Autodesk Inventor part; units mm, degrees
ref_plane "YZ Plane" through (0, 0, 0) normal (1, 0, 0) x (0, 1, 0)
ref_plane "XZ Plane" through (0, 0, 0) normal (0, 1, 0) x (-1, 0, 0)
ref_plane "XY Plane" through (0, 0, 0) normal (0, 0, 1) x (1, 0, 0)
sketch "Sketch1" plane through (0, 0, 0) normal (0, 0, 1) x (1, 0, 0)
  arc A0 (-5.217, 1.3451) -> (-5.1032, 1.1142) centre (-4.8204, 1.397) ccw
  line L0 (-5.1032, 1.1142) -> (-4.8872, 0.8982)
  arc A1 (-4.77, 0.6153) -> (-4.8872, 0.8982) centre (-5.17, 0.6153) ccw
  line L1 (-4.77, 0.6153) -> (-4.77, -0.9467)
  arc A2 (-4.8872, -1.2296) -> (-4.77, -0.9467) centre (-5.17, -0.9467) ccw
  line L2 (-4.8872, -1.2296) -> (-7.2071, -3.5495)
  arc A3 (-7.2071, -3.5495) -> (-7.5, -4.2566) centre (-6.5, -4.2566) ccw
  line L3 (-7.5, -4.2566) -> (-7.5, -6.8)
  line L4 (-7.5, -6.8) -> (-6.8, -7.5)
  line L5 (-6.8, -7.5) -> (6.8, -7.5)
  line L6 (6.8, -7.5) -> (7.5, -6.8)
  line L7 (7.5, -6.8) -> (7.5, -4.2566)
  arc A4 (7.5, -4.2566) -> (7.2071, -3.5495) centre (6.5, -4.2566) ccw
  line L8 (7.2071, -3.5495) -> (4.8872, -1.2296)
  arc A5 (4.77, -0.9467) -> (4.8872, -1.2296) centre (5.17, -0.9467) ccw
  line L9 (4.77, -0.9467) -> (4.77, 0.6153)
  arc A6 (4.8872, 0.8982) -> (4.77, 0.6153) centre (5.17, 0.6153) ccw
  line L10 (4.8872, 0.8982) -> (5.1032, 1.1142)
  arc A7 (5.1032, 1.1142) -> (5.217, 1.3451) centre (4.8204, 1.397) ccw
  arc A8 (6.7419, 2.7529) -> (5.217, 1.3451) centre (6.8233, 1.1349) ccw
  line L11 (6.7419, 2.7529) -> (7.5, 3.511)
  line L12 (7.5, 3.511) -> (7.5, 5.049)
  line L13 (7.5, 5.049) -> (6.7304, 5.8186)
  arc A9 (5.2183, 7.2157) -> (6.7304, 5.8186) centre (6.8233, 7.436) ccw
  arc A10 (5.2183, 7.2157) -> (5.1049, 7.4441) centre (4.822, 7.1613) ccw
  line L14 (5.1049, 7.4441) -> (5.049, 7.5)
  line L15 (5.049, 7.5) -> (-5.049, 7.5)
  line L16 (-5.049, 7.5) -> (-5.1049, 7.4441)
  arc A11 (-5.1049, 7.4441) -> (-5.2183, 7.2157) centre (-4.822, 7.1613) ccw
  arc A12 (-6.7304, 5.8186) -> (-5.2183, 7.2157) centre (-6.8233, 7.436) ccw
  line L17 (-6.7304, 5.8186) -> (-7.5, 5.049)
  line L18 (-7.5, 5.049) -> (-7.5, 3.511)
  line L19 (-7.5, 3.511) -> (-6.7419, 2.7529)
  arc A13 (-5.217, 1.3451) -> (-6.7419, 2.7529) centre (-6.8233, 1.1349) ccw
  line L20 (-7.5, -5.5283) -> (-10, -5.5283)
  line L21 (-10, -5.5283) -> (-10, 14.2)
  line L22 (-10, 14.2) -> (10, 14.2)
  line L23 (10, 14.2) -> (10, -5.5283)
  line L24 (10, -5.5283) -> (7.5, -5.5283)
  arc A14 (-7.2778, -3.4788) -> (-7.6, -4.2566) centre (-6.5, -4.2566) ccw
  line L25 (-7.2778, -3.4788) -> (-4.9579, -1.1589)
  arc A15 (-4.9579, -1.1589) -> (-4.87, -0.9467) centre (-5.17, -0.9467) ccw
  line L26 (-4.87, -0.9467) -> (-4.87, 0.6153)
  arc A16 (-4.87, 0.6153) -> (-4.9579, 0.8275) centre (-5.17, 0.6153) ccw
  line L27 (-4.9579, 0.8275) -> (-5.1739, 1.0435)
  arc A17 (-5.3161, 1.3322) -> (-5.1739, 1.0435) centre (-4.8204, 1.397) ccw
  arc A18 (-5.3161, 1.3322) -> (-6.7848, 2.6544) centre (-6.8233, 1.1349) ccw
  line L28 (-6.7848, 2.6544) -> (-7.6, 3.4696)
  line L29 (-7.6, 3.4696) -> (-7.6, 5.0904)
  line L30 (-7.6, 5.0904) -> (-6.7736, 5.9168)
  arc A19 (-6.7736, 5.9168) -> (-5.3174, 7.2293) centre (-6.8233, 7.436) ccw
  arc A20 (-5.1756, 7.5148) -> (-5.3174, 7.2293) centre (-4.822, 7.1613) ccw
  line L31 (-5.1756, 7.5148) -> (-5.0904, 7.6)
  line L32 (-5.0904, 7.6) -> (5.0904, 7.6)
  line L33 (5.0904, 7.6) -> (5.1756, 7.5148)
  arc A21 (5.3174, 7.2293) -> (5.1756, 7.5148) centre (4.822, 7.1613) ccw
  arc A22 (5.3174, 7.2293) -> (6.7736, 5.9168) centre (6.8233, 7.436) ccw
  line L34 (6.7736, 5.9168) -> (7.6, 5.0904)
  line L35 (7.6, 5.0904) -> (7.6, 3.4696)
  line L36 (7.6, 3.4696) -> (6.7848, 2.6544)
  arc A23 (6.7848, 2.6544) -> (5.3161, 1.3322) centre (6.8233, 1.1349) ccw
  arc A24 (5.1739, 1.0435) -> (5.3161, 1.3322) centre (4.8204, 1.397) ccw
  line L37 (5.1739, 1.0435) -> (4.9579, 0.8275)
  arc A25 (4.9579, 0.8275) -> (4.87, 0.6153) centre (5.17, 0.6153) ccw
  line L38 (4.87, 0.6153) -> (4.87, -0.9467)
  arc A26 (4.87, -0.9467) -> (4.9579, -1.1589) centre (5.17, -0.9467) ccw
  line L39 (4.9579, -1.1589) -> (7.2778, -3.4788)
  arc A27 (7.6, -4.2566) -> (7.2778, -3.4788) centre (6.5, -4.2566) ccw
  line L40 (7.6, -4.2566) -> (7.6, -6.8414)
  line L41 (7.6, -6.8414) -> (6.8414, -7.6)
  line L42 (6.8414, -7.6) -> (-6.8414, -7.6)
  line L43 (-6.8414, -7.6) -> (-7.6, -6.8414)
  line L44 (-7.6, -6.8414) -> (-7.6, -4.2566)
  point P0 (0, 0)
  point P1 (-7.6, -5.5283)
  point P2 (7.6, -5.5283)
  dimension "d2" = 6.7
  dimension "d20" = 2.5
  dimension "d21" = 0.1
extrude "Extrusion1" add sketch "Sketch1" against normal blind 15 contours L20 L21 L22 L23 L24 L40 A27 L39 A26 L38 A25 L37 A24 A23 L36 L35 L34 A22 A21 L33 L32 L31 A20 A19 L30 L29 L28 A18 A17 L27 A16 L26 A15 L25 A14 L44
chamfer "Chamfer1" distance 1.5 angle 45 10 edges at (-10, -5.5283, -7.5) (-10, 4.3358, -15) (-10, 4.3358, 0) (0, 14.2, -15) (0, 14.2, 0) (-10, 14.2, -7.5) (10, 4.3358, -15) (10, 4.3358, 0) (10, -5.5283, -7.5) (10, 14.2, -7.5)
sketch "Sketch3" plane through (-5.049, 7.6, 0) normal (0, -1, 0) x (1, 0, 0)
  line L0 (5.049, 0) -> (5.049, -15) construction
  circle A0 centre (5.049, -7.5) radius 2.65
  line L1 (10.1394, -15) -> (-0.0414, -15)
  dimension "d8" = 5.3
extrude "Extrusion2" cut sketch "Sketch3" against normal blind 15
sketch "Sketch4" plane through (-5.049, 7.6, 0) normal (0, -1, 0) x (1, 0, 0)
  line L0 (1.049, -5.1906) -> (5.049, -2.8812)
  line L1 (5.049, -2.8812) -> (9.049, -5.1906)
  line L2 (9.049, -5.1906) -> (9.049, -9.8094)
  line L3 (9.049, -9.8094) -> (5.049, -12.1188)
  line L4 (5.049, -12.1188) -> (1.049, -9.8094)
  line L5 (1.049, -9.8094) -> (1.049, -5.1906)
  point P0 (5.049, 0)
  point P1 (5.049, -7.5)
  point P2 (5.049, -7.5)
  dimension "d11" = 8
extrude "Extrusion3" cut sketch "Sketch4" against normal blind 4
sketch "Sketch5" plane through (10, -4.0283, -13.5) normal (1, 0, 0) x (0, 0, -1)
  line L0 (0, 0) -> (-12, 0)
  line L1 (0, 16.7283) -> (0, 0)
  line L2 (-12, 16.7283) -> (0, 16.7283)
  line L3 (-12, 0) -> (-12, 16.7283)
  line L4 (-10.5, 15.2283) -> (-1.5, 15.2283)
  line L5 (-1.5, 15.2283) -> (-1.5, 1.5)
  line L6 (-1.5, 1.5) -> (-10.5, 1.5)
  line L7 (-10.5, 1.5) -> (-10.5, 15.2283)
  point P0 (-13.5, 4.0283)
  dimension "d14" = 1.5
extrude "Extrusion4" cut sketch "Sketch5" against normal blind 1.5 contours L4 L5 L6 L7
chamfer "Chamfer2" distance 1.5 angle 45 4 edges at (8.5, 4.3358, -3) (8.5, -2.5283, -7.5) (8.5, 11.2, -7.5) (8.5, 4.3358, -12)
mirror "Mirror1" about plane through (0, 0, 0) normal (1, 0, 0) of "Extrusion4", "Chamfer2"
properties part number "Tope Final" material "PET Plastic"
Geometry: final body of the model. Coordinates: model frame, mm. A direction names the side the tool comes from. Round coordinates to 2 decimals unless told otherwise and drop trailing zeros. Write each loop counter-clockwise with the first axis right and the second up, starting at its lowest first coordinate (ties: lowest second). Pieces come first, ordered by that corner, then holes.
Item 1: Section query A-A (y = -3). Return loops of the section in (x, z).
Item 2: Material intervals for L1, parallel to X at y = -1, z = -6.5; L2, parallel to Y at x = 3.25, z = -6.75; L3, parallel to Z at x = 0, y = 13.15, sorted ascending.
Item 3: Mould query, pull axis Z, two halves, no side actions, for faces 5 (the face through (-8, -5.528, -7)), 6 (the face through (9.073, 13.153, -1.026)), 7 (the face through (8.5, 4, -7)), 8 (the face through (9, 4, -4)). Classes: +Z half, -Z half, draft (parallel to the pull), parting line (faces both ways), or undercut.
Item 4: Section query B-B (x = -6). Return loops of the section in (y, z), plus the area to 3 significant figures.
Item 5: Pin query (flat end, axial travel): P1, Ø0.6, axis at y = -5, z = -6.5, coming from the -X side; P2, Ø6.5, axis at y = 3.5, z = -8, coming from the +X side; P3, Ø8.5, axis at x = 0, z = -7.5, coming from the -Y side. Return the tip coordinate at first contact, or that it passes through.
Item 6: Set-up query: faces 1 (the face through (4.87, 0, -7)), 2 (the face through (5.818, 2.275, -7.395)), 3 (the face through (9.2, 10.4, -7.4)), 4 (the face through (-9, 4, -11)). Return all of +Z, -Z, +X, -X, +Y, -Y with unobstructed straight access to the full face (end or side cutting, diameter ignored); none if empty.
Item 7: Section query C-C (x = 1). Return loops of the section in (y, z).
Completed:
1. outline: (-10, -13.5) - (-8.5, -15) - (-6.8, -15) - (-6.8, 0) - (-8.5, 0) - (-10, -1.5) - close; (6.8, -15) - (8.5, -15) - (10, -13.5) - (10, -1.5) - (8.5, 0) - (6.8, 0) - close
2. L1: x = -8.5 to -4.87, 4.87 to 8.5
2. L2: y = 11.6 to 14.2
2. L3: z = -14.55 to -10.15, -4.85 to -0.45
3. face 5: draft
3. face 6: +Z half
3. face 7: undercut
3. face 8: undercut
4. outline: (-2.2, -15) - (2.41, -15) - (2.41, 0) - (-2.2, 0) - close; (6.16, -15) - (12.7, -15) - (14.2, -13.5) - (14.2, -1.5) - (12.7, 0) - (6.16, 0) - close
4. area: 188 mm2
5. P1: stops at x = -9.33
5. P2: stops at x = 9.25
5. P3: stops at y = 7.6
6. face 1: +Z, -Z, -Y
6. face 2: +Z, -Z
6. face 3: +X
6. face 4: -X
7. outline: (7.6, -15) - (12.7, -15) - (14.2, -13.5) - (14.2, -9.95) - (11.6, -9.95) - (11.6, -11.54) - (7.6, -11.54) - close; (7.6, -3.46) - (11.6, -3.46) - (11.6, -5.05) - (14.2, -5.05) - (14.2, -1.5) - (12.7, 0) - (7.6, 0) - close
